Design review of the part built by this model. Coordinates are the model's own, in mm. Face numbers are marked on the shaded views. A direction names the side the tool comes from. Coordinates: 2 decimals unless noted, no trailing zeros. Loops run counter-clockwise (first coordinate to the right, second up) from the corner with the lowest first, then second, coordinate; pieces in that order, holes last. Notation, with made-up numbers: M 83,16.5 L 142,16.5 A15 cw 142,23.5 Z; hole C -39.75,29.5 d4. An arc over 180 degrees is marked long. One line per item, written item: value.
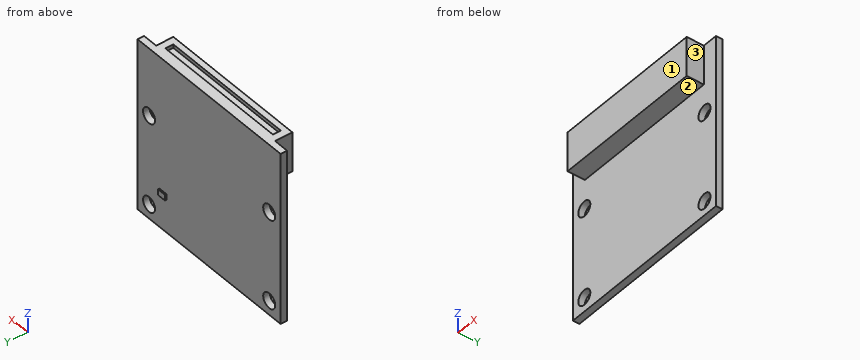
```python
from build123d import *

# Parameters (mm, degrees)
SKIZZE1_W               = 25
SKIZZE1_H               = 24
PCB_DEPTH               = 0.9
SKIZZE2_R               = 1.05
MOUNTING_HOLES_DEPTH    = 1.9
SKIZZE3_W               = 20.8
SKIZZE3_H               = 5.5
CONNECTOR_CLOSED_DEPTH  = 2.4
ESQUISSE1_W             = 1.22
ESQUISSE1_H             = 0.8
STATUS_LED_DEPTH        = 0.2
ESQUISSE3_W             = 18.8
ESQUISSE3_H             = 1.1
ENL_V_MAT_EXTRU_1_DEPTH = 0.5


with BuildPart() as part:
    # Skizze1 → PCB (new body)
    with BuildSketch(Plane(origin=(0, 0, 0), x_dir=(1, 0, 0), z_dir=(0, 1, 0))):
        with Locations((0, 2.5)):
            Rectangle(SKIZZE1_W, SKIZZE1_H)
    extrude(amount=-PCB_DEPTH)

    # Skizze2 → Mounting_Holes (cut, through all)
    with BuildSketch(Plane(origin=(0, 0, 0), x_dir=(1, 0, 0), z_dir=(0, 1, 0))):
        with Locations((10.5, 12.5)):
            Circle(SKIZZE2_R)
        with Locations((10.5, 0)):
            Circle(SKIZZE2_R)
        with Locations((-10.5, 0)):
            Circle(SKIZZE2_R)
        with Locations((-10.5, 12.5)):
            Circle(SKIZZE2_R)
    extrude(amount=-MOUNTING_HOLES_DEPTH, mode=Mode.SUBTRACT)

    # Skizze3 → Connector_closed (add)
    with BuildSketch(Plane.XZ.offset(0.9)):
        with Locations((0, 6.75)):
            Rectangle(SKIZZE3_W, SKIZZE3_H)
    extrude(amount=CONNECTOR_CLOSED_DEPTH)

    # Esquisse1 → Status LED (add)
    with BuildSketch(Plane(origin=(0, 0, 0), x_dir=(1, 0, 0), z_dir=(0, 1, 0))):
        with Locations((8.09, 9.5)):
            Rectangle(ESQUISSE1_W, ESQUISSE1_H)
    extrude(amount=STATUS_LED_DEPTH)

    # Esquisse3 → Enlèv. mat.-Extru.1 (cut)
    with BuildSketch(Plane.XY.offset(9.5)):
        with Locations((0, -1.95)):
            Rectangle(ESQUISSE3_W, ESQUISSE3_H)
    extrude(amount=-ENL_V_MAT_EXTRU_1_DEPTH, mode=Mode.SUBTRACT)


solid = part.part
```
(1) We need section C-C on x = -6.75. State the section outline as (y, z) points.
Reply:
outline: M -3.3,4 L -0.9,4 L -0.9,-14.5 L 0,-14.5 L 0,9.5 L -1.4,9.5 L -1.4,9 L -2.5,9 L -2.5,9.5 L -3.3,9.5 Z
(2) Insertion check: pin 1 (1.9 mm diameter, centred on y = -2.5, z = 6.5, fed in from -X); pin 2 (1.2 mm diameter, centred on y = -2, z = 7.5, fed in from +X); pin 3 (12 mm diameter, centred on x = -5, z = -7.5, fed in from +Y). Each pin has a flat end and moves straight along its axis. Give the tip position at first contact, or say it passes through.
Reply:
pin 1: stops at x = -10.4
pin 2: stops at x = 10.4
pin 3: stops at y = 0
(3) We need section B-B on y = -0.6. State the section outline as (x, z) points, then the cut area to 3 significant figures.
Reply:
outline: M -12.5,-14.5 L 12.5,-14.5 L 12.5,9.5 L -12.5,9.5 Z; hole C -10.5,-12.5 d2.1; hole C -10.5,0 d2.1; hole C 10.5,-12.5 d2.1; hole C 10.5,0 d2.1
area: 586 mm2
(4) Tool access review of the marked faces 1, 2 and 3: name each direction out of +Z, -Z, +X, -X, +Y, -Y from which nothing blocks a thin tool from reaching the whole face with its end or side.
Reply:
face 1: +Z, -Z, +X, -X, -Y
face 2: -Z, +X, -X, -Y
face 3: +Z, -Z, +X, -Y
(5) We need section A-A on z = 0. State the section outline as (x, y) points.
Reply:
outline: M -12.5,-0.9 L -11.55,-0.9 L -11.55,0 L -12.5,0 Z; M -9.45,-0.9 L 9.45,-0.9 L 9.45,0 L -9.45,0 Z; M 11.55,-0.9 L 12.5,-0.9 L 12.5,0 L 11.55,0 Z
(6) To check wall thickness, follow line 1 along Z through (x, y) = (10.5, -0.65); line 2 along Y through (x, z) = (10.5, -2.5); line 3 along X through (y, z) = (-3, 7.25). State the ranges of each line that lie inside material, in increasing order. Write a range as [from, to].
Reply:
line 1: z = [-14.5, -13.55], [-11.45, -1.05], [1.05, 9.5]
line 2: y = [-0.9, 0]
line 3: x = [-10.4, 10.4]
(7) We need section D-D on z = -4. State the section outline as (x, y) points.
Reply:
outline: M -12.5,-0.9 L 12.5,-0.9 L 12.5,0 L -12.5,0 Z
